Part model, mm, in its own coordinate system. Face numbers are marked on the shaded views. A direction names the side the tool comes from. Give positions to 0.01 mm unless a question says otherwise; leave off trailing zeros. Write each loop counter-clockwise with the first axis right and the second up, starting at its lowest first coordinate (ties: lowest second). Pieces come first, ordered by that corner, then holes. Notation, with made-up numbers: (50, 71) - (78, 71) arc R19 cw to (78, 88) - close; hole circle Ø4 at (-16, 72). An arc over 180 degrees is marked (long way). Answer in a Markdown table with one row per item. Add a question column.
1. Probe line 1 along Z through (x, y) = (-3.5, -17); line 2 along Y through (x, z) = (-15.5, 8); line 3 along X through (y, z) = (-24.75, 0). List the from-to ranges inside material, lowest first.
2. Drop flat-ended pins along their axis: pin 1 Ø1.5 at (x, y) = (11.5, -20) entering from +Z; pin 2 Ø2 at (y, z) = (-5.5, -7.5) entering from -X; pin 3 Ø10 at (x, y) = (-9.5, -22) entering from +Z. Give the stop position or say it passes through.
3. Band-saw the part on D-D on z = 10. Write the cut outline in (x, y), plus the area to 3 significant figures.
4. Band-saw the part on C-C on y = -23. Write the cut outline in (x, z).
5. Which spindle directions (+Z, -Z, +X, -X, +Y, -Y) get a long thin tool onto all of the face, cutting with end or side? Do the marked faces 5, 6, 7 and 8. Say none if no direction does.
6. Band-saw the part on B-B on x = 0. Write the cut outline in (y, z), plus the area to 3 significant figures.
7. Pull direction Y, two halves, no side cores. Call the marked faces 1, 2, 3 and 4: released by +Y, released by -Y, zero draft, split by the parting line, or undercut.
8. Band-saw the part on A-A on z = 16. Write the cut outline in (x, y), plus the area to 3 significant figures.
```python
from build123d import *

# Parameters (mm, degrees)
EXTRUDE_3_DEPTH     = 18
SKETCH_2_R          = 1.8
CUT_EXTRUDE_1_DEPTH = 17.325
SKETCH_4_R          = 20
SKETCH_4_R_2        = 1.75
EXTRUDE_4_DEPTH     = 3
SKETCH_5_R          = 15
SKETCH_5_R_2        = 1.75
EXTRUDE_5_DEPTH     = 8
SKETCH_6_R          = 20
SKETCH_6_R_2        = 1.75
EXTRUDE_6_DEPTH     = 3


with BuildPart() as part:
    # 草图1 → 凸台-拉伸3 (new body)
    with BuildSketch(Plane(origin=(0, 0, 0), x_dir=(1, 0, 0), z_dir=(0, 1, 0))):
        Polygon((10, 0), (5, 8.660254038), (-5, 8.660254038), (-10, 0), (-5, -8.660254038), (5, -8.660254038), align=None)
        Polygon((6.985938257, 0), (3.492969129, 6.05), (-3.492969129, 6.05), (-6.985938257, 0), (-3.492969129, -6.05), (3.492969129, -6.05), align=None, mode=Mode.SUBTRACT)
    extrude(amount=-EXTRUDE_3_DEPTH)

    # 草图2 → 切除-拉伸1 (cut)
    with BuildSketch(Plane(origin=(7.5, 0, -4.330127019), x_dir=(-0.5000000000000003, 0, -0.8660254037844386), z_dir=(0.8660254037844386, 0, -0.5000000000000003))):
        with Locations((0, -4.5)):
            Circle(SKETCH_2_R)
    extrude(amount=-CUT_EXTRUDE_1_DEPTH, mode=Mode.SUBTRACT)

    # 草图4 → 凸台-拉伸4 (add)
    with BuildSketch(Plane.XZ.offset(18)):
        with Locations(Location((0, 0, 0), (0, 0, 270))):
            Circle(SKETCH_4_R)
        with Locations(Location((0, 0, 0), (0, 0, 270))):
            Circle(SKETCH_4_R_2, mode=Mode.SUBTRACT)
    extrude(amount=EXTRUDE_4_DEPTH)

    # 草图5 → 凸台-拉伸5 (add)
    with BuildSketch(Plane.XZ.offset(21)):
        with Locations(Location((0, 0, 0), (0, 0, 270))):
            Circle(SKETCH_5_R)
        with Locations(Location((0, 0, 0), (0, 0, 270))):
            Circle(SKETCH_5_R_2, mode=Mode.SUBTRACT)
    extrude(amount=EXTRUDE_5_DEPTH)

    # 草图6 → 凸台-拉伸6 (add)
    with BuildSketch(Plane.XZ.offset(29)):
        with Locations(Location((0, 0, 0), (0, 0, 270))):
            Circle(SKETCH_6_R)
        with Locations(Location((0, 0, 0), (0, 0, 270))):
            Circle(SKETCH_6_R_2, mode=Mode.SUBTRACT)
    extrude(amount=EXTRUDE_6_DEPTH)


solid = part.part
```
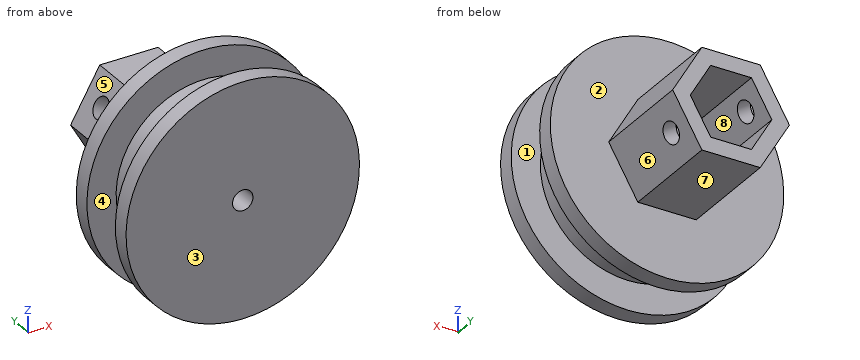
Values:
| question | item | result |
|---|---|---|
| 1 | line 1 | z = -8.66 to -6.04, 6.04 to 8.66 |
| 1 | line 2 | y = -32 to -29, -21 to -18 |
| 1 | line 3 | x = -15 to -1.75, 1.75 to 15 |
| 2 | pin 1 | stops at z = 16.87 |
| 2 | pin 2 | stops at x = -6.25 |
| 2 | pin 3 | stops at z = 19.46 |
| 3 | outline | (-17.32, -32) - (17.32, -32) - (17.32, -29) - (11.18, -29) - (11.18, -21) - (17.32, -21) - (17.32, -18) - (-17.32, -18) - (-17.32, -21) - (-11.18, -21) - (-11.18, -29) - (-17.32, -29) - close |
| 3 | area | 387 mm² |
| 4 | outline | circle Ø30 at (0, 0); hole circle Ø3.5 at (0, 0) |
| 5 | face 5 | +Z, -X, +Y |
| 5 | face 6 | -Z, +X, +Y |
| 5 | face 7 | -Z, +X, -X, +Y |
| 5 | face 8 | +Y |
| 6 | outline | (-32, -20) - (-29, -20) - (-29, -15) - (-21, -15) - (-21, -20) - (-18, -20) - (-18, -8.66) - (0, -8.66) - (0, -6.05) - (-18, -6.05) - (-18, -1.75) - (-32, -1.75) - close; (-32, 1.75) - (-18, 1.75) - (-18, 6.05) - (0, 6.05) - (0, 8.66) - (-18, 8.66) - (-18, 20) - (-21, 20) - (-21, 15) - (-29, 15) - (-29, 20) - (-32, 20) - close |
| 6 | area | 525 mm² |
| 7 | face 1 | undercut |
| 7 | face 2 | released by +Y |
| 7 | face 3 | released by -Y |
| 7 | face 4 | undercut |
| 8 | outline | (-12, -32) - (12, -32) - (12, -29) - (-12, -29) - close; (-12, -21) - (12, -21) - (12, -18) - (-12, -18) - close |
| 8 | area | 144 mm² |
